```python
from build123d import *

# Parameters (mm, degrees)
SKETCH_1_R          = 30
EXTRUDE_1_DEPTH     = 8
SKETCH_2_R          = 2.75
CUT_EXTRUDE_1_DEPTH = 50
SKETCH_3_R          = 2.75
CUT_EXTRUDE_2_DEPTH = 20
SKETCH_4_R          = 2.75
CUT_EXTRUDE_3_DEPTH = 10


with BuildPart() as part:
    # 草图1 → 凸台-拉伸1 (new body)
    with BuildSketch(Plane.XY):
        with BuildLine():
            Line((-48, 114), (-48, 0))
            Line((-48, 0), (48, 0))
            Line((48, 0), (48, 114))
            ThreePointArc((48, 114), (0, 150), (-48, 114))
        make_face()
        with Locations((0, 100)):
            Circle(SKETCH_1_R, mode=Mode.SUBTRACT)
    extrude(amount=EXTRUDE_1_DEPTH)

    # 草图2 → 切除-拉伸1 (cut)
    with BuildSketch(Plane.XZ):
        with Locations(Location((35, 4, 0), (0, 0, 270))):
            Circle(SKETCH_2_R)
        with Locations(Location((-35, 4, 0), (0, 0, 270))):
            Circle(SKETCH_2_R)
    extrude(amount=-CUT_EXTRUDE_1_DEPTH, mode=Mode.SUBTRACT)

    # 草图3 → 切除-拉伸2 (cut)
    with BuildSketch(Plane.XY.offset(8)):
        with Locations((0, 40)):
            Circle(SKETCH_3_R)
    extrude(amount=-CUT_EXTRUDE_2_DEPTH, mode=Mode.SUBTRACT)

    # 草图4 → 切除-拉伸3 (cut)
    with BuildSketch(Plane.XY.offset(8)):
        with Locations((9.058666579, 133.80740392)):
            Circle(SKETCH_4_R)
        with Locations((24.748737342, 124.748737342)):
            Circle(SKETCH_4_R)
        with Locations((33.80740392, 109.058666579)):
            Circle(SKETCH_4_R)
        with Locations((33.80740392, 90.941333421)):
            Circle(SKETCH_4_R)
        with Locations((24.748737342, 75.251262658)):
            Circle(SKETCH_4_R)
        with Locations((9.058666579, 66.19259608)):
            Circle(SKETCH_4_R)
        with Locations((-9.058666579, 66.19259608)):
            Circle(SKETCH_4_R)
        with Locations((-24.748737342, 75.251262658)):
            Circle(SKETCH_4_R)
        with Locations((-33.80740392, 90.941333421)):
            Circle(SKETCH_4_R)
        with Locations((-33.80740392, 109.058666579)):
            Circle(SKETCH_4_R)
        with Locations((-24.748737342, 124.748737342)):
            Circle(SKETCH_4_R)
        with Locations((-9.058666579, 133.80740392)):
            Circle(SKETCH_4_R)
    extrude(amount=-CUT_EXTRUDE_3_DEPTH, mode=Mode.SUBTRACT)


solid = part.part
```
Geometry: final body of the model. Coordinates: model frame, mm. A direction names the side the tool comes from. Round coordinates to 2 decimals unless told otherwise and drop trailing zeros. Order: outer loops, then holes, each group sorted by start corner. A loop starts at its lowest first (then second) coordinate and runs counter-clockwise, first axis right, second up. Notation, with made-up numbers: (45, 80) - (104, 80) arc R29 cw to (104, 113) - close; hole circle Ø10 at (80, 47.25). An arc over 180 degrees is marked (long way). Use CSV: the item, a comma, the result in double quotes. Start each with the question number.
Q1. Section query B-B (y = 100). Return loops of the section in (x, z).
Q2. Section query A-A (y = 40). Return loops of the section in (x, z), and give its area (3 significant figures).
Q3. Access query for faces 5 (the face through (-34.165, 111.785, 4.056)), 6 (the face through (35, 50, 4)). Directions: +Z, -Z, +X, -X, +Y, -Y. A direction counts if a zero-diameter tool reaches every point of the face in a straight line with its end or side. Return the directions, or none.
Q4. First-contact query: pin 1 (3.5 mm diameter, centred on x = 9.06, y = 133.81, fed in from -Z) (3 decimals); pin 2 (4.5 mm diameter, centred on x = -35, z = 4, fed in from +Y); pin 3 (3 mm diameter, centred on x = 24.5, z = 1, fed in from +Y). Flat tips, straight axial feed; report the tip coordinate or a pass-through.
Q5. Section query D-D (x = 35). Return loops of the section in (y, z), and give its area (3 significant figures).
Q6. Section query C-C (z = 5.5). State how many separate pieces and enclosed holes the cut face has, and give its area (3 significant figures).
Q7. Mould query, pull axis Y, two halves, no side actions, for faces 1 (the face through (33.449, 111.785, 4.056)), 2 (the face through (-34.404, 88.257, 4.056)), 3 (the face through (-35, 50, 4)), 4 (the face through (-1, 59, 8)). Classes: +Y half, -Y half, draft (parallel to the pull), parting line (faces both ways), or undercut.
Q8. Material intervals for line 1 along X through (y, z) = (43, 3.75); line 2 along Y through (x, z) = (0, 4.25); line 3 along X through (y, z) = (34, 4.75), sorted ascending. Write a range as from..to.
Result set:
1,outline,"(-48, 0) - (-30, 0) - (-30, 8) - (-48, 8) - close; (30, 0) - (48, 0) - (48, 8) - (30, 8) - close"
2,outline,"(-48, 0) - (-2.75, 0) - (-2.75, 8) - (-48, 8) - close; (2.75, 0) - (48, 0) - (48, 8) - (2.75, 8) - close; hole circle Ø5.5 at (-35, 4); hole circle Ø5.5 at (35, 4)"
2,area,"676 mm2"
3,face 5,"+Z, -Z"
3,face 6,"-Y"
4,pin 1,"passes through"
4,pin 2,"stops at y = 137.78"
4,pin 3,"stops at y = 144.4"
5,outline,"(0, 0) - (88.46, 0) - (88.46, 8) - (0, 8) - (0, 6.75) - (50, 6.75) - (50, 1.25) - (0, 1.25) - close; (93.42, 0) - (106.58, 0) - (106.58, 8) - (93.42, 8) - close; (111.54, 0) - (135.71, 0) - (135.71, 8) - (111.54, 8) - close"
5,area,"731 mm2"
6,separate pieces,"1"
6,enclosed holes,"14"
6,area,"9,890 mm2"
7,face 1,"undercut"
7,face 2,"undercut"
7,face 3,"-Y half"
7,face 4,"draft"
8,line 1,"x = -48..-37.74, -32.26..32.26, 37.74..48"
8,line 2,"y = 0..37.25, 42.75..70, 130..150"
8,line 3,"x = -48..-37.65, -32.35..32.35, 37.65..48"
